Check sheet for the modelled part. Datum: model origin and axes. Units: mm. A direction names the side the tool comes from. Coordinates: 2 decimals unless noted, no trailing zeros. Write each loop counter-clockwise with the first axis right and the second up, starting at its lowest first coordinate (ties: lowest second). Pieces come first, ordered by that corner, then holes. Notation, with made-up numbers: (59.5, 2) -> (86.5, 2) arc R23 ccw to (86.5, 17) -> close; hole circle Ø2 at (-34, 60.25). An arc over 180 degrees is marked (long way). One line per item, written item: value. Start each with the question number.
1) Sectioned sample at C-C on z = 20. Enter the section's corners in (x, y).
2) Scan lines: line 1 along Y through (x, z) = (5, 0.5); line 2 along X through (y, z) = (20.5, -89); line 3 along Z through (x, y) = (15, -78.5). Record each from-to range of solid material in increasing order. Write a range as [from, to].
3) Sectioned sample at A-A on z = -60.5. Enter the section's corners in (x, y), plus the area to 3 significant figures.
4) Set-up check for faces 5 (the flat face through (20, -63, 32)), 6 (the flat face through (-30.3, -17.3, -26)), 7 (the flat face through (0, -63, -36)), 8 (the flat face through (0, -93.5, -24)), 9 (the flat face through (-27, -20, 32)): record each of +Z, -Z, +X, -X, +Y, -Y from which the full face is reachable in a straight line by a thin tool's end or side.
5) Draft check along Y on faces 1 (the flat face through (-31.479, 2.925, 20.137)), 2 (the flat face through (30, -57, 32)), 3 (the flat face through (18, -63, -41)), 4 (the flat face through (33, -98, -27)). Enter one of: +Y half, -Y half, draft (parallel to the pull), parting line (faces both ways), or undercut.
6) Sectioned sample at B-B on y = -36. Enter the section's corners in (x, z).
7) Sectioned sample at D-D on x = 3. Enter the section's corners in (y, z).
8) Gauge pin test, flat ends, axial feed: P1, Ø2.5, axis at x = -31, y = 4, coming from the +Z side; P2, Ø10, axis at x = 2.5, y = -43.5, coming from the +Z side; P3, Ø5, axis at y = -59, z = -41.5, coming from the +X side; P4, Ø1.5, axis at y = -28.5, z = -9, coming from the -X side. Record the tip position at first contact, or that the pin passes through.
```python
from build123d import *

# Parameters (mm, degrees)
SKETCH_1_W      = 60
SKETCH_1_H      = 3
EXTRUDE_1_DEPTH = 65
SKETCH_2_W      = 40
SKETCH_2_H      = 3.5
EXTRUDE_2_DEPTH = 46
EXTRUDE_3_DEPTH = 3.5
SKETCH_5_W      = 35
SKETCH_5_H      = 17
EXTRUDE_4_DEPTH = 3
EXTRUDE_START   = 3
SKETCH_6_W      = 35
SKETCH_6_H      = 17
SKETCH_6_W_2    = 20
SKETCH_6_H_2    = 3.5
EXTRUDE_5_DEPTH = 3
SKETCH_7_W      = 36
SKETCH_7_H      = 10
SKETCH_7_W_2    = 10
SKETCH_7_H_2    = 65
EXTRUDE_6_DEPTH = 60
SKETCH_8_W      = 66
SKETCH_8_H      = 111
EXTRUDE_7_DEPTH = 10
SKETCH_9_W      = 15
SKETCH_9_H      = 10
EXTRUDE_8_DEPTH = 70


with BuildPart() as part:
    # 草图1 → 凸台-拉伸1 (new body)
    with BuildSketch(Plane.XY):
        with Locations((0, -32)):
            Rectangle(SKETCH_1_W, SKETCH_1_H)
        with BuildLine():
            Line((-20, -24), (-20, -28))
            Line((-20, -28), (-20, -30))
            Line((-20, -30), (20, -30))
            Line((20, -30), (20, -28))
            Line((20, -28), (20, -24))
            ThreePointArc((20, -24), (21.171572875, -21.171572875), (24, -20))
            Line((24, -20), (28, -20))
            Line((28, -20), (30, -20))
            Line((30, -20), (30, -30.5))
            Line((30, -30.5), (-30, -30.5))
            Line((-30, -30.5), (-30, -20))
            Line((-30, -20), (-28, -20))
            Line((-28, -20), (-24, -20))
            ThreePointArc((-24, -20), (-21.171572875, -21.171572875), (-20, -24))
        make_face()
    extrude(amount=EXTRUDE_1_DEPTH)

    # 草图2 → 凸台-拉伸2 (add)
    with BuildSketch(Plane(origin=(0, 0, 0), x_dir=(-1, 0, 0), z_dir=(0, 0, -1))):
        with Locations((0, -31.75)):
            Rectangle(SKETCH_2_W, SKETCH_2_H)
    extrude(amount=EXTRUDE_2_DEPTH)

    # 草图4 → 凸台-拉伸3 (add)
    with BuildSketch(Plane.XZ.offset(33.5)):
        Polygon((20, -46), (30, -46), (30, -26), (20, -26), (-30, -26), (-30, -46), align=None)
    extrude(amount=-EXTRUDE_3_DEPTH)

    # 草图5 → 凸台-拉伸4 (add)
    with BuildSketch(Plane.ZY.offset(30)):
        with BuildLine():
            Line((-46, -26.5), (-46, -33.5))
            Line((-46, -33.5), (-26, -33.5))
            Line((-26, -33.5), (-26, 8.5))
            Line((-26, 8.5), (56.193548387, -33.5))
            Line((56.193548387, -33.5), (65, -20))
            Line((65, -20), (-26, 26.5))
            Line((-26, 26.5), (-96, 26.5))
            ThreePointArc((-96, 26.5), (-105, 17.5), (-96, 8.5))
            Line((-96, 8.5), (-96, -8.5))
            ThreePointArc((-96, -8.5), (-105, -17.5), (-96, -26.5))
            Line((-96, -26.5), (-46, -26.5))
        make_face()
        with Locations((-63.5, 0)):
            Rectangle(SKETCH_5_W, SKETCH_5_H, mode=Mode.SUBTRACT)
    extrude(amount=EXTRUDE_4_DEPTH)

    # 草图6 → 凸台-拉伸5 (add)
    # profile 1 of 3: a face of its own
    with BuildSketch(Plane(origin=(30, 0, 0), x_dir=(0, 0, -1), z_dir=(1, 0, 0)).offset(EXTRUDE_START)):
        Polygon((26, 8.5), (26, 26.5), (-65, -20), (-56.193548387, -33.5), align=None)
    # profile 2 of 3: a face of its own
    with BuildSketch(Plane(origin=(30, 0, 0), x_dir=(0, 0, -1), z_dir=(1, 0, 0)).offset(EXTRUDE_START)):
        with BuildLine():
            Line((96, 26.5), (46, 26.5))
            Line((46, 26.5), (26, 26.5))
            Line((26, 26.5), (26, 8.5))
            Line((26, 8.5), (26, -30))
            Line((26, -30), (46, -30))
            Line((46, -30), (46, -26.5))
            Line((46, -26.5), (96, -26.5))
            ThreePointArc((96, -26.5), (105, -17.5), (96, -8.5))
            Line((96, -8.5), (96, 8.5))
            ThreePointArc((96, 8.5), (105, 17.5), (96, 26.5))
        make_face()
        with Locations((63.5, 0)):
            Rectangle(SKETCH_6_W, SKETCH_6_H, mode=Mode.SUBTRACT)
    # profile 3 of 3: a face of its own
    with BuildSketch(Plane(origin=(30, 0, 0), x_dir=(0, 0, -1), z_dir=(1, 0, 0)).offset(EXTRUDE_START)):
        with Locations((36, -31.75)):
            Rectangle(SKETCH_6_W_2, SKETCH_6_H_2)
    extrude(amount=-EXTRUDE_5_DEPTH)

    # 草图7 → 凸台-拉伸6 (add)
    with BuildSketch(Plane.XZ.offset(33.5)):
        with Locations((0, -41)):
            Rectangle(SKETCH_7_W, SKETCH_7_H)
        with Locations((-25, 32.5)):
            Rectangle(SKETCH_7_W_2, SKETCH_7_H_2)
        with Locations((25, 32.5)):
            Rectangle(SKETCH_7_W_2, SKETCH_7_H_2)
    extrude(amount=EXTRUDE_6_DEPTH)

    # 草图8 → 凸台-拉伸7 (add)
    with BuildSketch(Plane.XZ.offset(93.5)):
        with Locations((0, 9.5)):
            Rectangle(SKETCH_8_W, SKETCH_8_H)
    extrude(amount=EXTRUDE_7_DEPTH)

    # 草图9 → 凸台-拉伸8 (add)
    with BuildSketch(Plane(origin=(0, 0, -46), x_dir=(-1, 0, 0), z_dir=(0, 0, -1))):
        with Locations((25.5, -98.5)):
            Rectangle(SKETCH_9_W, SKETCH_9_H)
        with Locations((-25.5, -98.5)):
            Rectangle(SKETCH_9_W, SKETCH_9_H)
    extrude(amount=EXTRUDE_8_DEPTH)


solid = part.part
```
Answers:
1. outline: (-33, -103.5) -> (33, -103.5) -> (33, -93.5) -> (30, -93.5) -> (30, -20) -> (24, -20) arc R4 ccw to (20, -24) -> (20, -30) -> (-20, -30) -> (-20, -24) arc R4 ccw to (-24, -20) -> (-30, -20) -> (-30, -93.5) -> (-33, -93.5) -> close; (-33, -15.01) -> (-30, -15.01) -> (-30, 2.99) -> (-33, 2.99) -> close; (30, -15.01) -> (33, -15.01) -> (33, 2.99) -> (30, 2.99) -> close; hole (-20, -93.5) -> (20, -93.5) -> (20, -33.5) -> (-20, -33.5) -> close
2. line 1: y = [-103.5, -93.5], [-33.5, -30]
2. line 2: x = [-33, -30], [30, 33]
2. line 3: z = [-46, -36]
3. outline: (-33, -103.5) -> (-18, -103.5) -> (-18, -93.5) -> (-33, -93.5) -> close; (-33, -26.5) -> (-30, -26.5) -> (-30, -8.5) -> (-33, -8.5) -> close; (-33, 8.5) -> (-30, 8.5) -> (-30, 26.5) -> (-33, 26.5) -> close; (18, -103.5) -> (33, -103.5) -> (33, -93.5) -> (18, -93.5) -> close; (30, -26.5) -> (33, -26.5) -> (33, -8.5) -> (30, -8.5) -> close; (30, 8.5) -> (33, 8.5) -> (33, 26.5) -> (30, 26.5) -> close
3. area: 516 mm2
4. face 5: +Z, -Z
4. face 6: -X
4. face 7: +Z, +X, -X
4. face 8: none
4. face 9: +Z, -Z, +Y
5. face 1: +Y half
5. face 2: undercut
5. face 3: undercut
5. face 4: draft
6. outline: (-30, 0) -> (-20, 0) -> (-20, 65) -> (-30, 65) -> close; (-18, -46) -> (18, -46) -> (18, -36) -> (-18, -36) -> close; (20, 0) -> (30, 0) -> (30, 65) -> (20, 65) -> close
7. outline: (-103.5, -46) -> (-30, -46) -> (-30, 65) -> (-33.5, 65) -> (-33.5, -36) -> (-93.5, -36) -> (-93.5, 65) -> (-103.5, 65) -> close
8. P1: stops at z = 20.48
8. P2: stops at z = -36
8. P3: stops at x = 18
8. P4: passes through
